```python
from build123d import *
from build123d.topology import SkipClean

# Parameters (mm, degrees)
ESQUISSE2_R                 = 3.25
BOSS_EXTRU_3_DEPTH          = 2
BOSS_EXTRU_4_DEPTH          = 3.75
BOSS_EXTRU_5_DEPTH          = 1.15
TROU_TARAUD_M43_D           = 3.3
TROU_TARAUD_M43_CSINK_D     = 4.05
TROU_TARAUD_M43_CSINK_ANGLE = 90


with BuildPart() as part:
    # Esquisse2 → Boss.-Extru.3 (new, symmetric)
    with BuildSketch(Plane.XY):
        with BuildLine():
            Line((-8, 50.5), (8, 50.5))
            Line((8, 50.5), (15.610501, 42.889499))
            Line((15.610501, 42.889499), (7.011413, 19.263699))
            ThreePointArc((7.011413, 19.263699), (0, 20.5), (-7.011413, 19.263699))
            Line((-7.011413, 19.263699), (-15.610501, 42.889499))
            Line((-15.610501, 42.889499), (-8, 50.5))
        make_face()
        with Locations((0, 28.5)):
            Circle(ESQUISSE2_R, mode=Mode.SUBTRACT)
    extrude(amount=BOSS_EXTRU_3_DEPTH, both=True)

    # Esquisse3 → Boss.-Extru.4 (add, symmetric)
    with BuildSketch(Plane.XY.offset(2)):
        Polygon((15.610501, 42.889499), (8, 50.5), (-8, 50.5), (-15.610501, 42.889499), (-14.478369, 39.778991), (-6.757359, 47.5), (6.757359, 47.5), (14.478369, 39.778991), align=None)
    extrude(amount=BOSS_EXTRU_4_DEPTH, both=True)

    # Esquisse4 → Boss.-Extru.5 (add, symmetric)
    with SkipClean():  # the faces are left unmerged after this step: merging them gives an invalid solid
        with BuildSketch(Plane.XY.offset(2)):
            with BuildLine():
                Line((8.593256, 23.609777), (10.901892, 29.952702))
                ThreePointArc((10.901892, 29.952702), (6.272313, 31.251779), (1.5, 31.839686))
                Line((1.5, 31.839686), (1.5, 31.383141))
                ThreePointArc((1.5, 31.383141), (3.25, 28.5), (1.5, 25.616859))
                Line((1.5, 25.616859), (1.5, 25.080184))
                ThreePointArc((1.5, 25.080184), (5.0999, 24.601964), (8.593256, 23.609777))
            make_face()
            with BuildLine():
                Line((-10.901892, 29.952702), (-8.593256, 23.609777))
                ThreePointArc((-8.593256, 23.609777), (-5.0999, 24.601964), (-1.5, 25.080184))
                Line((-1.5, 25.080184), (-1.5, 25.616859))
                ThreePointArc((-1.5, 25.616859), (-3.25, 28.5), (-1.5, 31.383141))
                Line((-1.5, 31.383141), (-1.5, 31.839686))
                ThreePointArc((-1.5, 31.839686), (-6.272313, 31.251779), (-10.901892, 29.952702))
            make_face()
        extrude(amount=BOSS_EXTRU_5_DEPTH, both=True)

    # Trou taraudé M43 (through all)
    with Locations(Plane.XY.offset(2)):
        with Locations((-6, 39.772078), (6, 39.772078)):
            CounterSinkHole(TROU_TARAUD_M43_D / 2, TROU_TARAUD_M43_CSINK_D / 2, counter_sink_angle=TROU_TARAUD_M43_CSINK_ANGLE)


solid = part.part
```
CAD build for the part. Positions are in the model's coordinates, mm. A direction names the side the tool comes from. Give positions to 0.01 mm unless a question says otherwise; leave off trailing zeros. Order: outer loops, then holes, each group sorted by start corner. A loop starts at its lowest first (then second) coordinate and runs counter-clockwise, first axis right, second up. Notation, with made-up numbers: M -39,5.25 L 7,5.25 A23 ccw 7,24.25 Z; hole C 75,1 d7. An arc over 180 degrees is marked long. Put each result on its own line as item: value. Start each with the question number.
(1) Saw through at B-B, the plane y = 28.5. Write the cut outline in (x, z), then the cut area to 3 significant figures.
(2) Which spindle directions (+Z, -Z, +X, -X, +Y, -Y) get a long thin tool onto all of the face, cutting with end or side? Do faces 1 (the cylindrical face through (-5.1, 24.6, 2.6)), 2 (the cylindrical face through (6.34, 31.24, 2.57)), 3 (the flat face through (-10.67, 43.59, 3.9)). Say none if no direction does.
(3) Drill centre lines: line 1 along Z through (x, y) = (10.5, 41.5); line 2 along Z through (x, y) = (-5, 29.5); line 3 along Y through (x, z) = (-6, -1.2). Where is each one in solid material? Low to high.
(4) Saw through at D-D, the plane z = 1.25. Write the cut outline in (x, y).
(5) Saw through at C-C, the plane z = 5. Write the cut outline in (x, y).
(6) Saw through at A-A, the plane x = 0. Write the cut outline in (y, z), then the cut area to 3 significant figures.
(7) Flat gauge pins, fed straight in: pin 1 Ø4 at (x, y) = (-4, 27) entering from +Z; pin 2 Ø1.5 at (x, y) = (-2, 34) entering from +Z; pin 3 Ø7.5 at (x, y) = (0, 28.5) entering from -Z; pin 4 Ø1 at (x, z) = (-3, 1.5) entering from -Y. Where does each tip first touch, or does it go through?
(8) Mould opens along Z. For faces 4 (the flat face through (6, 28, 3.15)), 5 (the flat face through (0, 35, -2)), 6 (the cylindrical face through (-4.69, 38.77, -0.21)) say: +Z half, -Z half, draft (parallel to the pull), parting line (faces both ways), or undercut.
Check result:
1. outline: M -10.37,-2 L -3.25,-2 L -3.25,3.15 L -10.37,3.15 Z; M 3.25,-2 L 10.37,-2 L 10.37,3.15 L 3.25,3.15 Z
1. area: 73.4 mm2
2. face 1: +Z, -Y
2. face 2: +Z, +X
2. face 3: +Z
3. line 1: z = -2 to 2
3. line 2: z = -2 to 3.15
3. line 3: y = 19.6 to 38.12, 41.42 to 50.5
4. outline: M -15.61,42.89 L -7.01,19.26 A20.5 cw 7.01,19.26 L 15.61,42.89 L 8,50.5 L -8,50.5 Z; hole C -6,39.77 d3.3; hole C 0,28.5 d6.5; hole C 6,39.77 d3.3
5. outline: M -15.61,42.89 L -14.48,39.78 L -6.76,47.5 L 6.76,47.5 L 14.48,39.78 L 15.61,42.89 L 8,50.5 L -8,50.5 Z
6. outline: M 20.5,-2 L 25.25,-2 L 25.25,2 L 20.5,2 Z; M 31.75,-2 L 50.5,-2 L 50.5,5.75 L 47.5,5.75 L 47.5,2 L 31.75,2 Z
6. area: 105 mm2
7. pin 1: stops at z = 3.15
7. pin 2: stops at z = 2
7. pin 3: stops at z = -2
7. pin 4: stops at y = 20.2
8. face 4: +Z half
8. face 5: -Z half
8. face 6: draft
